from build123d import *

# Parameters (mm, degrees)
F1_DEPTH = 4.064
F2_R     = 3.048
F3_DEPTH = 18.796
F4_SIZE  = 0.254


with BuildPart() as f1:
    # F0 (on Front) → F1 (new body)
    with BuildSketch(Plane.XZ):
        Polygon((3.182239, 5.5118), (-3.182239, 5.5118), (-6.364478, 0), (-3.182239, -5.5118), (3.182239, -5.5118), (6.364478, 0), align=None)
    extrude(amount=F1_DEPTH)

    # F2 (on face) → F3 (join)
    with BuildSketch(Plane(origin=(0, 0, 0), x_dir=(-1, 0, 0), z_dir=(0, 1, 0))):
        Circle(F2_R)
    extrude(amount=F3_DEPTH)

    # F4
    f4_edges = [f1.edges().sort_by_distance(p)[0] for p in [
        (3.048, 18.796, 0),
    ]]
    chamfer(f4_edges, length=F4_SIZE)


solid = f1.part
The listing builds one solid part. Answer for the finished solid, in the listing's coordinates (mm). A direction names the side the tool comes from. Give positions to 0.01 mm unless a question says otherwise; leave off trailing zeros. Write each loop counter-clockwise with the first axis right and the second up, starting at its lowest first coordinate (ties: lowest second). Pieces come first, ordered by that corner, then holes.
Item 1: Section D-D, the plane z = -5 is taken. Write down the section's boundary in (x, y).
Item 2: Find the intervals of material crossed by line 1 along Y through (x, z) = (-2.75, 2.5); line 2 along X through (y, z) = (14.25, -2); line 3 along X through (y, z) = (8, 1), in increasing order.
Item 3: Which of the six approach directions +Z, -Z, +X, -X, +Y, -Y give full straight-line access (tool end or side, diameter ignored) to faces 1 (the cylindrical face through (0.4, 9.14, 3.02)), 2 (the flat face through (0, -4.064, 0))?
Item 4: Flat-ended cylindrical pins translate along their axes: P1, Ø4, axis at x = -0.5, y = 5, coming from the -Z side; P2, Ø1, axis at y = 2, z = -0.5, coming from the +X side; P3, Ø1.5, axis at y = 9.5, z = -1, coming from the -X side. Find the tip coordinate at first contact, or state that the pin passes through.
Item 5: Section B-B, the plane y = -1.75 is taken. Write down the section's boundary in (x, z), plus the area to 3 significant figures.
Item 6: Section C-C, the plane y = 6.5 is taken. Write down the section's boundary in (x, z).
Item 7: Section A-A, the plane x = 0 is taken. Write down the section's boundary in (y, z), plus the area to 3 significant figures.
Completed:
1. outline: (-3.48, -4.06) - (3.48, -4.06) - (3.48, 0) - (-3.48, 0) - close
2. line 1: y = -4.06 to 0
2. line 2: x = -2.3 to 2.3
2. line 3: x = -2.88 to 2.88
3. face 1: +Y
3. face 2: +Z, -Z, +X, -X, -Y
4. P1: stops at z = -3.05
4. P2: stops at x = 3.05
4. P3: stops at x = -3.04
5. outline: (-6.36, 0) - (-3.18, -5.51) - (3.18, -5.51) - (6.36, 0) - (3.18, 5.51) - (-3.18, 5.51) - close
5. area: 105 mm2
6. outline: circle Ø6.1 at (0, 0)
7. outline: (-4.06, -5.51) - (0, -5.51) - (0, -3.05) - (18.54, -3.05) - (18.8, -2.79) - (18.8, 2.79) - (18.54, 3.05) - (0, 3.05) - (0, 5.51) - (-4.06, 5.51) - close
7. area: 159 mm2
